from build123d import *

# Parameters (mm, degrees)
F0_W     = 152.4
F0_H     = 152.4
F1_DEPTH = 152.4
F2_W     = 34.9075235426
F2_H     = 33.3854667842
F2_W_2   = 35.112304613
F2_H_2   = 9.2097893357
F2_W_3   = 58.1367611885
F2_H_3   = 10.9366215765
F2_W_4   = 8.0585666001
F2_H_4   = 63.3172709495
F2_W_5   = 44.897697866
F2_H_5   = 64.4684825093
F2_W_6   = 27.629353106
F2_H_6   = 60.4392085224
F2_W_7   = 31.0830175877
F2_H_7   = 11.5122310817
F2_W_8   = 65.0440976024
F2_H_8   = 32.2342440486
F2_W_9   = 8.6341686547
F2_H_9   = 8.6341649294
F2_W_10  = 14.9659141898
F2_H_10  = 44.8977053165
F2_W_11  = 4.6048909426
F2_H_11  = 35.1123064756
F2_W_12  = 23.0244547129
F2_H_12  = 37.9903591238
F2_W_13  = 13.239055872
F2_H_13  = 61.5904331207
F2_W_14  = 31.0830101371
F2_H_14  = 29.3561927974
F2_W_15  = 14.3903046846
F2_H_15  = 25.9025096893
F2_W_16  = 72.5270435214
F2_H_16  = 11.5122199059
F2_W_17  = 36.2635287456
F2_H_17  = 20.1463997364
F3_DEPTH = 25.4
F4_DEPTH = 50.8


with BuildPart() as f1:
    # F0 (on Top) → F1 (new body)
    with BuildSketch(Plane.XY):
        Rectangle(F0_W, F0_H)
    extrude(amount=F1_DEPTH)

    # F2 (on face) → F3 (join)
    with BuildSketch(Plane.XY.offset(152.4)):
        Rectangle(F2_W, F2_H)
        with Locations((2.4878596887, -25.0390991569)):
            Rectangle(F2_W_2, F2_H_2)
        with Locations((17.4537617713, 25.6147123873)):
            Rectangle(F2_W_3, F2_H_3)
        with Locations((-25.1414887607, 28.7805777043)):
            Rectangle(F2_W_4, F2_H_4)
        with Locations((-43.8488647342, -41.4440259337)):
            Rectangle(F2_W_5, F2_H_5)
        with Locations((-51.0440096259, 39.4293889403)):
            Rectangle(F2_W_6, F2_H_6)
        with Locations((-49.6049784124, 0)):
            Rectangle(F2_W_7, F2_H_7)
        with Locations((17.4537617713, 50.9416200221)):
            Rectangle(F2_W_8, F2_H_8)
        with Locations((-25.1414887607, 68.4977695346)):
            Rectangle(F2_W_9, F2_H_9)
        with Locations((66.0929381847, 46.3367253542)):
            Rectangle(F2_W_10, F2_H_10)
        with Locations((53.4294769168, 11.2244244665)):
            Rectangle(F2_W_11, F2_H_11)
        with Locations((36.44894436, -2.3024461698)):
            Rectangle(F2_W_12, F2_H_12)
        with Locations((66.3807466626, -11.2244244665)):
            Rectangle(F2_W_13, F2_H_13)
        with Locations((40.1904173195, -41.1562249064)):
            Rectangle(F2_W_14, F2_H_14)
        with Locations((66.9563561678, -61.0148198903)):
            Rectangle(F2_W_15, F2_H_15)
        with Locations((19.4684006274, -66.4831325412)):
            Rectangle(F2_W_16, F2_H_16)
        with Locations((2.7756656054, -44.897697866)):
            Rectangle(F2_W_17, F2_H_17)
    extrude(amount=F3_DEPTH)

    # F4 (cut): faces of the model
    f4_faces = [f1.faces().sort_by_distance(p)[0] for p in [
        (-51.0440096259, 39.4293889403, 177.8),
        (0, 0, 177.8),
        (40.1904173195, -41.1562249064, 177.8),
        (-43.8488647342, -41.4440259337, 177.8),
        (66.0929381847, 46.3367253542, 177.8),
        (-25.1414887607, 68.4977695346, 177.8),
        (53.4294769168, 11.2244244665, 177.8),
    ]]
    extrude(f4_faces, amount=-F4_DEPTH, mode=Mode.SUBTRACT)


solid = f1.part
Source: CAD feature listing. Evaluate the final solid. Frame: model axes, mm. A direction names the side the tool comes from. Round coordinates to 2 decimals unless told otherwise and drop trailing zeros. Loops run counter-clockwise (first coordinate to the right, second up) from the corner with the lowest first, then second, coordinate; pieces in that order, holes last. Notation, with made-up numbers: M -20,81.25 L 21,81.25 A16 ccw 21,97.25 Z; hole C -1,51 d3. An arc over 180 degrees is marked long. Return JSON: item names as keys, results as strings. Group by question number.
1. Material intervals for line 1 along Y through (x, z) = (-10, 158.5); line 2 along Y through (x, z) = (39, 158.5); line 3 along Y through (x, z) = (-57, 148.5), sorted ascending. Write a range as from..to.
2. Section query A-A on z = 145.5. State how many separate pieces and enclosed holes the cut face has, and give its area (3 significant figures).
3. Section query D-D on x = -53.5. Output: boundary loops of the cut face in (y, z).
4. Mould query, pull axis Y, two halves, no side actions, for faces 1 (the face through (-15.068, -25, 165)), 2 (the face through (17.454, 0, 140)), 3 (the face through (19, -72.239, 165)). Classes: released by +Y, released by -Y, zero draft, split by the parting line, or undercut.
5. Section query B-B on x = 38.5. Output: boundary loops of the cut face in (y, z), and give its area (3 significant figures).
6. Pin query (flat end, axial travel): pin 1 (2 mm diameter, centred on y = 26.5, z = 159, fed in from +X); pin 2 (7.5 mm diameter, centred on x = 13.5, z = 160.5, fed in from -Y); pin 3 (3 mm diameter, centred on y = -44, z = 154, fed in from +X). Return the tip coordinate at first contact, or that it passes through.
7. Section query C-C on y = -64.5. Output: boundary loops of the cut face in (x, z), and give its area (3 significant figures).
8. Reachability of faces 4 (the face through (2, -20.434, 165)), 5 (the face through (67, -48.064, 165)), 6 (the face through (-25, 64.181, 140)) from +Z, -Z, +X, -X, +Y, -Y: full face, straight path, thin tool, end or side. Return the list, or none.
Checks:
{
 "1": {"line 1": "y = -72.24..-60.73, -54.97..-34.82, -29.64..-20.43, 20.15..31.08, 34.82..67.06", "line 2": "y = -72.24..-60.73, -21.3..16.69, 20.15..31.08, 34.82..67.06", "line 3": "y = -76.2..-73.68, -9.21..9.21, 69.65..76.2"},
 "2": {"separate pieces": "1", "enclosed holes": "7", "area": "15,700 mm²"},
 "3": {"outline": "M -76.2,0 L 76.2,0 L 76.2,152.4 L 69.65,152.4 L 69.65,127 L 9.21,127 L 9.21,152.4 L 5.76,152.4 L 5.76,177.8 L -5.76,177.8 L -5.76,152.4 L -9.21,152.4 L -9.21,127 L -73.68,127 L -73.68,152.4 L -76.2,152.4 Z"},
 "4": {"face 1": "zero draft", "face 2": "undercut", "face 3": "released by -Y"},
 "5": {"outline": "M -76.2,0 L 76.2,0 L 76.2,152.4 L 67.06,152.4 L 67.06,177.8 L 34.82,177.8 L 34.82,152.4 L 31.08,152.4 L 31.08,177.8 L 20.15,177.8 L 20.15,152.4 L 16.69,152.4 L 16.69,177.8 L -21.3,177.8 L -21.3,152.4 L -26.48,152.4 L -26.48,127 L -55.83,127 L -55.83,152.4 L -60.73,152.4 L -60.73,177.8 L -72.24,177.8 L -72.24,152.4 L -76.2,152.4 Z", "area": "24,800 mm²"},
 "6": {"pin 1": "stops at x = 46.52", "pin 2": "stops at y = -72.24", "pin 3": "stops at x = 20.91"},
 "7": {"outline": "M -76.2,0 L 76.2,0 L 76.2,152.4 L 74.15,152.4 L 74.15,177.8 L 59.76,177.8 L 59.76,152.4 L 55.73,152.4 L 55.73,177.8 L -16.8,177.8 L -16.8,152.4 L -21.4,152.4 L -21.4,127 L -66.3,127 L -66.3,152.4 L -76.2,152.4 Z", "area": "24,300 mm²"},
 "8": {"face 4": "+Z, -X", "face 5": "+Z, +X", "face 6": "+Z"}
}
